The model under review builds one solid part; all positions refer to its coordinate system, in mm. Face numbers are marked on the shaded views. A direction names the side the tool comes from. Give positions to 0.01 mm unless a question says otherwise; leave off trailing zeros. Order: outer loops, then holes, each group sorted by start corner. A loop starts at its lowest first (then second) coordinate and runs counter-clockwise, first axis right, second up. Notation, with made-up numbers: (49, -7) - (77, -7) arc R10 cw to (77, 12) - close; hole circle Ø9 at (-5, -6). An arc over 180 degrees is marked (long way). Put each result on its own line as item: value.
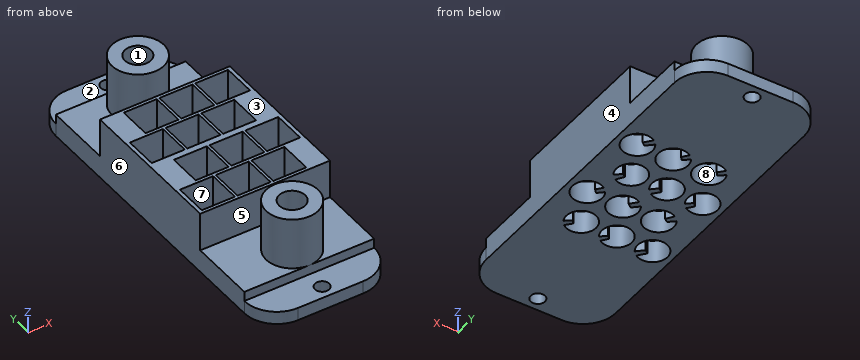
```python
from build123d import *

# Parameters (mm, degrees)
SKETCH013_W               = 20
SKETCH013_H               = 6
PAD013_DEPTH              = 2
SKETCH009_W               = 20
SKETCH009_H               = 27
SKETCH009_R               = 2.3
SKETCH009_R_2             = 1.1
PAD009_DEPTH              = 3.5
SKETCH010_W               = 20
SKETCH010_H               = 11.7
SKETCH010_W_2             = 5.1
SKETCH010_H_2             = 5.1
PAD010_DEPTH              = 6
SKETCH011_R               = 4
SKETCH011_R_2             = 2
PAD011_DEPTH              = 8
PAD012_DEPTH              = 3
FUSION001_PLACEMENT_ANGLE = 180
SKETCH_W                  = 20
SKETCH_H                  = 27
SKETCH_R                  = 2.3
SKETCH_R_2                = 1.1
PAD_DEPTH                 = 3.5
SKETCH001_W               = 20
SKETCH001_H               = 11.7
SKETCH001_W_2             = 5.1
SKETCH001_H_2             = 5.1
PAD001_DEPTH              = 6
SKETCH002_R               = 4
SKETCH002_R_2             = 2
PAD002_DEPTH              = 8
PAD003_DEPTH              = 3
FILLET_R                  = 5


with BuildPart() as pad013:
    # Sketch013 → Pad013 (new body)
    with BuildSketch(Plane.XY.offset(2)):
        with Locations((10, 25)):
            Rectangle(SKETCH013_W, SKETCH013_H)
        with Locations((10, -25)):
            Rectangle(SKETCH013_W, SKETCH013_H)
    extrude(amount=PAD013_DEPTH)


with BuildPart() as pad009:
    # Sketch009 → Pad009 (new body)
    with BuildSketch(Plane.XY):
        with Locations((10, 13.5)):
            Rectangle(SKETCH009_W, SKETCH009_H)
        with Locations((5.875, 8.65)):
            Circle(SKETCH009_R, mode=Mode.SUBTRACT)
        with Locations((11.375, 8.65)):
            Circle(SKETCH009_R, mode=Mode.SUBTRACT)
        with Locations((16.875, 8.65)):
            Circle(SKETCH009_R, mode=Mode.SUBTRACT)
        with Locations((14.125, 3.05)):
            Circle(SKETCH009_R, mode=Mode.SUBTRACT)
        with Locations((8.625, 3.05)):
            Circle(SKETCH009_R, mode=Mode.SUBTRACT)
        with Locations((3.125, 3.05)):
            Circle(SKETCH009_R, mode=Mode.SUBTRACT)
        with Locations((10, 25)):
            Circle(SKETCH009_R_2, mode=Mode.SUBTRACT)
    extrude(amount=PAD009_DEPTH)


with BuildPart() as pad010:
    # Sketch010 → Pad010 (new body)
    with BuildSketch(Plane.XY.offset(3.5)):
        with Locations((10, 5.85)):
            Rectangle(SKETCH010_W, SKETCH010_H)
        with Locations((5.875, 8.65)):
            Rectangle(SKETCH010_W_2, SKETCH010_H_2, mode=Mode.SUBTRACT)
        with Locations((11.375, 8.65)):
            Rectangle(SKETCH010_W_2, SKETCH010_H_2, mode=Mode.SUBTRACT)
        with Locations((16.875, 8.65)):
            Rectangle(SKETCH010_W_2, SKETCH010_H_2, mode=Mode.SUBTRACT)
        with Locations((3.125, 3.05)):
            Rectangle(SKETCH010_W_2, SKETCH010_H_2, mode=Mode.SUBTRACT)
        with Locations((8.625, 3.05)):
            Rectangle(SKETCH010_W_2, SKETCH010_H_2, mode=Mode.SUBTRACT)
        with Locations((14.125, 3.05)):
            Rectangle(SKETCH010_W_2, SKETCH010_H_2, mode=Mode.SUBTRACT)
    extrude(amount=PAD010_DEPTH)


with BuildPart() as pad011:
    # Sketch011 → Pad011 (new body)
    with BuildSketch(Plane.XY.offset(3.5)):
        with Locations((10, 18)):
            Circle(SKETCH011_R)
        with Locations((10, 18)):
            Circle(SKETCH011_R_2, mode=Mode.SUBTRACT)
    extrude(amount=PAD011_DEPTH)


with BuildPart() as fusion001:
    # Sketch012 → Pad012 (new body)
    with BuildSketch(Plane.XY):
        Polygon((3.14451, 10.296382), (4.812228, 8.962195), (5.229761, 9.506803), (3.848642, 11.027596), align=None)
        Polygon((8.80602, 10.523404), (10.348319, 9.131856), (10.816751, 9.610404), (9.51401, 11.285856), align=None)
        Polygon((14.379175, 10.541558), (16.031153, 8.980349), (16.575762, 9.434188), (15.141627, 11.176934), align=None)
        Polygon((3.671404, 2.070844), (4.913085, 0.518744), (5.689134, 1.228275), (4.18138, 2.602993), align=None)
        Polygon((8.904199, 2.181709), (10.38978, 0.496571), (11.121485, 1.250448), (9.547212, 2.669512), align=None)
        Polygon((14.558277, 2.181709), (15.66692, 0.518744), (16.553833, 1.33914), (15.090425, 2.602993), align=None)
    extrude(amount=PAD012_DEPTH)

    # Fusion001: union Pad009, Pad010, Pad011
    add(pad009.part)
    add(pad010.part)
    add(pad011.part)


with BuildPart() as fusion001_1:
    # Fusion001 placement: moved
    add(fusion001.part.moved(Location((20, 0, 0))).rotate(Axis((20, 0, 0), (0, 0, 1)), FUSION001_PLACEMENT_ANGLE))


with BuildPart() as pad:
    # Sketch → Pad (new body)
    with BuildSketch(Plane.XY):
        with Locations((10, 13.5)):
            Rectangle(SKETCH_W, SKETCH_H)
        with Locations((5.875, 8.65)):
            Circle(SKETCH_R, mode=Mode.SUBTRACT)
        with Locations((11.375, 8.65)):
            Circle(SKETCH_R, mode=Mode.SUBTRACT)
        with Locations((16.875, 8.65)):
            Circle(SKETCH_R, mode=Mode.SUBTRACT)
        with Locations((14.125, 3.05)):
            Circle(SKETCH_R, mode=Mode.SUBTRACT)
        with Locations((8.625, 3.05)):
            Circle(SKETCH_R, mode=Mode.SUBTRACT)
        with Locations((3.125, 3.05)):
            Circle(SKETCH_R, mode=Mode.SUBTRACT)
        with Locations((10, 25)):
            Circle(SKETCH_R_2, mode=Mode.SUBTRACT)
    extrude(amount=PAD_DEPTH)


with BuildPart() as pad001:
    # Sketch001 → Pad001 (new body)
    with BuildSketch(Plane.XY.offset(3.5)):
        with Locations((10, 5.85)):
            Rectangle(SKETCH001_W, SKETCH001_H)
        with Locations((5.875, 8.65)):
            Rectangle(SKETCH001_W_2, SKETCH001_H_2, mode=Mode.SUBTRACT)
        with Locations((11.375, 8.65)):
            Rectangle(SKETCH001_W_2, SKETCH001_H_2, mode=Mode.SUBTRACT)
        with Locations((16.875, 8.65)):
            Rectangle(SKETCH001_W_2, SKETCH001_H_2, mode=Mode.SUBTRACT)
        with Locations((3.125, 3.05)):
            Rectangle(SKETCH001_W_2, SKETCH001_H_2, mode=Mode.SUBTRACT)
        with Locations((8.625, 3.05)):
            Rectangle(SKETCH001_W_2, SKETCH001_H_2, mode=Mode.SUBTRACT)
        with Locations((14.125, 3.05)):
            Rectangle(SKETCH001_W_2, SKETCH001_H_2, mode=Mode.SUBTRACT)
    extrude(amount=PAD001_DEPTH)


with BuildPart() as pad002:
    # Sketch002 → Pad002 (new body)
    with BuildSketch(Plane.XY.offset(3.5)):
        with Locations((10, 18)):
            Circle(SKETCH002_R)
        with Locations((10, 18)):
            Circle(SKETCH002_R_2, mode=Mode.SUBTRACT)
    extrude(amount=PAD002_DEPTH)


with BuildPart() as cut:
    # Sketch003 → Pad003 (new body)
    with BuildSketch(Plane.XY):
        Polygon((3.14451, 10.296382), (4.812228, 8.962195), (5.229761, 9.506803), (3.848642, 11.027596), align=None)
        Polygon((8.80602, 10.523404), (10.348319, 9.131856), (10.816751, 9.610404), (9.51401, 11.285856), align=None)
        Polygon((14.379175, 10.541558), (16.031153, 8.980349), (16.575762, 9.434188), (15.141627, 11.176934), align=None)
        Polygon((3.671404, 2.070844), (4.913085, 0.518744), (5.689134, 1.228275), (4.18138, 2.602993), align=None)
        Polygon((8.904199, 2.181709), (10.38978, 0.496571), (11.121485, 1.250448), (9.547212, 2.669512), align=None)
        Polygon((14.558277, 2.181709), (15.66692, 0.518744), (16.553833, 1.33914), (15.090425, 2.602993), align=None)
    extrude(amount=PAD003_DEPTH)

    # Fusion: union Pad, Pad001, Pad002
    add(pad.part)
    add(pad001.part)
    add(pad002.part)

    # Fusion002: union Fusion001
    add(fusion001_1.part)

    # Fillet
    fillet_edges = [cut.edges().sort_by_distance(p)[0] for p in [
        (0, 27, 1.75),
        (20, 27, 1.75),
        (20, -27, 1.75),
        (0, -27, 1.75),
    ]]
    fillet(fillet_edges, radius=FILLET_R)

    # Cut: cut Pad013
    add(pad013.part, mode=Mode.SUBTRACT)


solid = cut.part
```
(1) For the marked faces 1, 2, 3 and 4, list the 3-axis set-ups (+Z, -Z, +X, -X, +Y, -Y) from which the entire face can be reached by the end or side of a thin tool; tool diameter is ignored.
The answers:
face 1: +Z
face 2: +Z, +X, -X, +Y
face 3: +Z, +X, -X
face 4: +Z, -Z, +X, +Y, -Y
(2) Take a section at C-C, the plane z = 8.25. Count the separate pieces of the cut face and the enclosed holes in it, then the cut area to 3 significant figures.
The answers:
separate pieces: 3
enclosed holes: 14
area: 231 mm^2
(3) Take a section at A-A, the plane y = -25. Write out the cut boundary in (x, z), then the cut area to 3 significant figures.
The answers:
outline: (1, 0) - (8.9, 0) - (8.9, 2) - (1, 2) - close; (11.1, 0) - (19, 0) - (19, 2) - (11.1, 2) - close
area: 31.6 mm^2
(4) Clearance check with flat-ended pins moving along their axes: pin 1 Ø1.6 at (x, y) = (15, 1.5) entering from +Z; pin 2 Ø2.5 at (x, z) = (8.5, 5.5) entering from +Y; pin 3 Ø4 at (y, z) = (-14.5, 7.5) entering from -X. State where each tip first meets the part, or that it passes through.
The answers:
pin 1: z = 3.5
pin 2: y = 21.99
pin 3: x = 6.29
(5) Wall thickness on L1, parallel to Y at x = 17, z = 5.25; L2, parallel to X at y = 8.65, z = 1.15 (3 decimals); L3, parallel to Y at x = 3.75, z = 8.25: over which ranges is each line inside the solid? List them lowest first.
The answers:
L1: -11.7 to -5.6, -0.5 to 6.1, 11.2 to 11.7
L2: 0 to 3.575, 8.175 to 9.075, 13.675 to 14.575, 19.175 to 20
L3: -11.7 to -11.2, -6.1 to -5.6, -0.5 to 0.5, 5.6 to 6.1, 11.2 to 11.7
(6) The part is to be moulded in two halves that separate along X. For the marked faces 5, 6, 7 and 8, say which applies: pulls with the +X half, pulls with the -X half, needs draft (parallel to the pull), parting line crosses it, or undercut.
The answers:
face 5: needs draft
face 6: pulls with the -X half
face 7: undercut
face 8: undercut
(7) Take a section at B-B, the plane x = 18.25. Write out the cut boundary in (y, z), then the cut area to 3 significant figures.
The answers:
outline: (-25.8, 0) - (-4.89, 0) - (-4.89, 3.5) - (-5.6, 3.5) - (-5.6, 9.5) - (-11.7, 9.5) - (-11.7, 3.5) - (-22, 3.5) - (-22, 2) - (-25.8, 2) - close; (-1.21, 0) - (6.81, 0) - (6.81, 3.5) - (6.1, 3.5) - (6.1, 9.5) - (-0.5, 9.5) - (-0.5, 3.5) - (-1.21, 3.5) - close; (10.49, 0) - (25.8, 0) - (25.8, 2) - (22, 2) - (22, 3.5) - (11.7, 3.5) - (11.7, 9.5) - (11.2, 9.5) - (11.2, 3.5) - (10.49, 3.5) - close
area: 223 mm^2
(8) Take a section at D-D, the plane y = 17. Write out the cut boundary in (x, z).
The answers:
outline: (0, 0) - (20, 0) - (20, 3.5) - (13.87, 3.5) - (13.87, 11.5) - (11.73, 11.5) - (11.73, 3.5) - (8.27, 3.5) - (8.27, 11.5) - (6.13, 11.5) - (6.13, 3.5) - (0, 3.5) - close
